Check sheet for the modelled part. Datum: model origin and axes. Units: mm. A direction names the side the tool comes from. Give positions to 0.01 mm unless a question says otherwise; leave off trailing zeros. Loops run counter-clockwise (first coordinate to the right, second up) from the corner with the lowest first, then second, coordinate; pieces in that order, holes last.
Autodesk Inventor part; units mm, degrees
ref_plane "YZ Plane" through (0, 0, 0) normal (1, 0, 0) x (0, 1, 0)
ref_plane "XZ Plane" through (0, 0, 0) normal (0, 1, 0) x (-1, 0, 0)
ref_plane "XY Plane" through (0, 0, 0) normal (0, 0, 1) x (1, 0, 0)
sketch "Sketch1" plane through (0, 0, 0) normal (0, 0, 1) x (1, 0, 0)
  point P0 (0, 0)
sketch "Sketch2" plane through (0, 0, 0) normal (0, 0, 1) x (1, 0, 0)
  line L0 (-11.4108, 7.8651) -> (12.0555, 7.8651)
  line L1 (12.0555, 7.8651) -> (12.0555, -8.2519)
  line L2 (12.0555, -8.2519) -> (-11.4108, -8.2519)
  line L3 (-11.4108, -8.2519) -> (-11.4108, 7.8651)
  point P0 (0, 0)
extrude "Extrusion1" add sketch "Sketch2" along normal blind 20.32
sketch "Sketch3" plane through (0, 0, 0) normal (0, 0, -1) x (-1, 0, 0)
  circle A0 centre (-8.9879, 0) radius 1.5322
  circle A1 centre (-4.3674, 0) radius 1.5722
  circle A2 centre (4.4307, 0) radius 1.5722
  circle A3 centre (8.7348, 0) radius 1.5671
  line L0 (-1.2026, 0.633) -> (1.2659, 0.633)
  line L1 (1.2659, 0.633) -> (1.2659, -1.1393)
  line L2 (1.2659, -1.1393) -> (-1.2026, -1.1393)
  line L3 (-1.2026, -1.1393) -> (-1.2026, 0.633)
  point P0 (0, 0)
extrude "Extrusion2" add sketch "Sketch3" along normal blind 2.54
sketch "Sketch4" plane through (-11.4108, 7.8651, 0) normal (0, 1, 0) x (1, 0, 0)
  circle A0 centre (11.7906, -10.8868) radius 4.4595
  point P0 (11.4108, 0)
extrude "Extrusion3" add sketch "Sketch4" along normal blind 3.81
properties part number "newcylinder1"
(1) Release check for a two-part mould opening along X. For faces 4 (the face through (12.056, 0, 10)), 5 (the face through (7.573, 0.587, -1.252)), 6 (the face through (-11.411, 0, 10)), 7 (the face through (0, -8.252, 10)) record: pulls with the +X half, pulls with the -X half, needs draft (parallel to the pull), parting line crosses it, or undercut.
(2) Section check D-D on x = 9.5. Record the boundary of the cut face in (y, z).
(3) Access from +Z, -Z, +X, -X, +Y, -Y to the whole of each face (thin tool, end or side, straight path). Record for faces 1 (the face through (-10.182, 0.6, -1.252)), 2 (the face through (-0.587, 9.743, 6.533)), 3 (the face through (0, 0.633, -1)).
(4) Material ranges on line 1 (Z direction, x = 0.5, y = 1.5); line 2 (Y direction, x = 5.75, z = 9); line 3 (X direction, y = 10, z = 13.5), recorded low to high.
(5) Section check A-A on y = 0. Record the boundary of the cut face in (x, z), plus the area to 3 significant figures.
(6) Section check B-B on x = 4. Record the boundary of the cut face in (y, z), plus the area to 3 significant figures.
(7) Gauge pin test, flat ends, axial feed: pin 1 Ø0.9 at (y, z) = (0, -2) entering from -X; pin 2 Ø1 at (x, z) = (-4, 6) entering from +Y; pin 3 Ø0.7 at (x, z) = (0, -2) entering from +Y. Record the tip position at first contact, or that the pin passes through.
(8) Section check C-C on z = 2. Record the boundary of the cut face in (x, y).
Computed values:
1. face 4: pulls with the +X half
1. face 5: undercut
1. face 6: pulls with the -X half
1. face 7: needs draft
2. outline: (-8.25, 0) - (-1.44, 0) - (-1.44, -2.54) - (1.44, -2.54) - (1.44, 0) - (7.87, 0) - (7.87, 20.32) - (-8.25, 20.32) - close
3. face 1: -Z
3. face 2: +Y
3. face 3: -Z, +Y
4. line 1: z = 0 to 20.32
4. line 2: y = -8.25 to 7.87
4. line 3: x = -3.23 to 3.99
5. outline: (-11.41, 0) - (-10.3, 0) - (-10.3, -2.54) - (-7.17, -2.54) - (-7.17, 0) - (-6, 0) - (-6, -2.54) - (-2.86, -2.54) - (-2.86, 0) - (-1.27, 0) - (-1.27, -2.54) - (1.2, -2.54) - (1.2, 0) - (2.8, 0) - (2.8, -2.54) - (5.94, -2.54) - (5.94, 0) - (7.46, 0) - (7.46, -2.54) - (10.52, -2.54) - (10.52, 0) - (12.06, 0) - (12.06, 20.32) - (-11.41, 20.32) - close
5. area: 515 mm2
6. outline: (-8.25, 0) - (-1.53, 0) - (-1.53, -2.54) - (1.53, -2.54) - (1.53, 0) - (7.87, 0) - (7.87, 8.28) - (11.68, 8.28) - (11.68, 13.49) - (7.87, 13.49) - (7.87, 20.32) - (-8.25, 20.32) - close
6. area: 355 mm2
7. pin 1: stops at x = -10.3
7. pin 2: stops at y = 7.87
7. pin 3: stops at y = 0.63
8. outline: (-11.41, -8.25) - (12.06, -8.25) - (12.06, 7.87) - (-11.41, 7.87) - close
